Model file for the job. Use its own axes, mm. Face numbers are marked on the shaded views. A direction names the side the tool comes from. Give positions to 0.01 mm unless a question says otherwise; leave off trailing zeros. Order: outer loops, then holes, each group sorted by start corner. A loop starts at its lowest first (then second) coordinate and runs counter-clockwise, first axis right, second up. Notation, with made-up numbers: M 52.25,40 L 98.25,40 A22 ccw 98.25,60 Z; hole C -27,60.5 d7. An arc over 180 degrees is marked long. Return JSON: item names as keys, results as strings. Group by question number.
1. 3-axis set-ups, long thin cutter, end or side, ignore diameter. For the marked faces 1 and 2: which of +Z, -Z, +X, -X, +Y, -Y reach the whole face in a straight line?
2. Slice it at D-D on y = -3.5. List the corners of the cut face in (x, z).
3. Wall check: probe 1 along Y at (x, z) = (-11.5, 4.5); probe 2 along Y at (x, z) = (11, 2); probe 3 along Z at (x, y) = (-13, -3.5). Give the ranges that are in metal, low to high. Write a range as [from, to].
4. Pin check, flat tips, straight feed: pin 1 (1.5 mm diameter, centred on x = -15, y = -6, fed in from +Z); pin 2 (1.5 mm diameter, centred on y = -10.5, z = 33, fed in from +X). Stop position of each tip, or through.
5. Slice it at B-B on z = 17.5. List the corners of the cut face in (x, y).
6. Slice it at C-C on x = -11.5. List the corners of the cut face in (y, z), then the cut area to 3 significant figures.
7. Two-plate mould, pull along Y, no slides. Class the marked faces 3, 4 and 5: released by +Y, released by -Y, zero draft, split by the parting line, or undercut.
8. Slice it at A-A on x = 0. List the corners of the cut face in (y, z), then the cut area to 3 significant figures.
from build123d import *

# Parameters (mm, degrees)
SKETCH_1_W      = 5
SKETCH_1_H      = 28
SKETCH_1_W_2    = 28
SKETCH_1_R      = 1.5
EXTRUDE_1_DEPTH = 10
SKETCH_3_W      = 10
SKETCH_3_H      = 28
SKETCH_3_W_2    = 5
EXTRUDE_3_DEPTH = 6
FILLET_3_R      = 5
FILLET_4_R      = 2


with BuildPart() as part:
    # 草图1 → 凸台-拉伸1 (new body)
    # profile 1 of 2: a face of its own
    with BuildSketch(Plane.XY):
        with Locations((-16.5, 0)):
            Rectangle(SKETCH_1_W, SKETCH_1_H)
    # profile 2 of 2: a face of its own
    with BuildSketch(Plane.XY):
        Rectangle(SKETCH_1_W_2, SKETCH_1_H)
        Circle(SKETCH_1_R, mode=Mode.SUBTRACT)
        with Locations((11.5, -11.5)):
            Circle(SKETCH_1_R, mode=Mode.SUBTRACT)
        with Locations((-11.5, -11.5)):
            Circle(SKETCH_1_R, mode=Mode.SUBTRACT)
        with Locations((11.5, 11.5)):
            Circle(SKETCH_1_R, mode=Mode.SUBTRACT)
        with Locations((-11.5, 11.5)):
            Circle(SKETCH_1_R, mode=Mode.SUBTRACT)
    extrude(amount=EXTRUDE_1_DEPTH)

    # 草图3 → 凸台-拉伸3 (add)
    with BuildSketch(Plane.ZY.offset(19)):
        with Locations((5, 0)):
            Rectangle(SKETCH_3_W, SKETCH_3_H)
        with Locations((12.5, 0)):
            Rectangle(SKETCH_3_W_2, SKETCH_3_H)
        with BuildLine():
            Line((16.616116524, 12.383883476), (15, 14))
            Line((15, 14), (15, -14))
            Line((15, -14), (16.616116524, -12.383883476))
            ThreePointArc((16.616116524, -12.383883476), (16.616116524, -10.616116524), (18.383883476, -10.616116524))
            Line((18.383883476, -10.616116524), (27.232233047, -1.767766953))
            ThreePointArc((27.232233047, -1.767766953), (26.5, 0), (27.232233047, 1.767766953))
            Line((27.232233047, 1.767766953), (18.383883476, 10.616116524))
            ThreePointArc((18.383883476, 10.616116524), (16.616116524, 10.616116524), (16.616116524, 12.383883476))
        make_face()
        with BuildLine():
            Line((43, 14), (15, 14))
            Line((15, 14), (16.616116524, 12.383883476))
            ThreePointArc((16.616116524, 12.383883476), (17.97835429, 12.654849416), (18.75, 11.5))
            ThreePointArc((18.75, 11.5), (18.654849416, 11.02164571), (18.383883476, 10.616116524))
            Line((18.383883476, 10.616116524), (27.232233047, 1.767766953))
            ThreePointArc((27.232233047, 1.767766953), (29, 2.5), (30.767766953, 1.767766953))
            Line((30.767766953, 1.767766953), (39.616116524, 10.616116524))
            ThreePointArc((39.616116524, 10.616116524), (39.616116524, 12.383883476), (41.383883476, 12.383883476))
            Line((41.383883476, 12.383883476), (43, 14))
        make_face()
        with BuildLine():
            Line((43, -14), (43, 14))
            Line((43, 14), (41.383883476, 12.383883476))
            ThreePointArc((41.383883476, 12.383883476), (41.654849416, 11.97835429), (41.75, 11.5))
            ThreePointArc((41.75, 11.5), (40.97835429, 10.345150584), (39.616116524, 10.616116524))
            Line((39.616116524, 10.616116524), (30.767766953, 1.767766953))
            ThreePointArc((30.767766953, 1.767766953), (31.309698831, 0.956708581), (31.5, 0))
            ThreePointArc((31.5, 0), (31.309698831, -0.956708581), (30.767766953, -1.767766953))
            Line((30.767766953, -1.767766953), (39.616116524, -10.616116524))
            ThreePointArc((39.616116524, -10.616116524), (40.97835429, -10.345150584), (41.75, -11.5))
            ThreePointArc((41.75, -11.5), (41.654849416, -11.97835429), (41.383883476, -12.383883476))
            Line((41.383883476, -12.383883476), (43, -14))
        make_face()
        with BuildLine():
            Line((16.616116524, -12.383883476), (15, -14))
            Line((15, -14), (43, -14))
            Line((43, -14), (41.383883476, -12.383883476))
            ThreePointArc((41.383883476, -12.383883476), (39.616116524, -12.383883476), (39.616116524, -10.616116524))
            Line((39.616116524, -10.616116524), (30.767766953, -1.767766953))
            ThreePointArc((30.767766953, -1.767766953), (29, -2.5), (27.232233047, -1.767766953))
            Line((27.232233047, -1.767766953), (18.383883476, -10.616116524))
            ThreePointArc((18.383883476, -10.616116524), (18.654849416, -11.02164571), (18.75, -11.5))
            ThreePointArc((18.75, -11.5), (17.97835429, -12.654849416), (16.616116524, -12.383883476))
        make_face()
    extrude(amount=EXTRUDE_3_DEPTH)

    # 圆角3
    fillet_3_edges = [part.edges().sort_by_distance(p)[0] for p in [
        (-25, 0, 0),
    ]]
    fillet(fillet_3_edges, radius=FILLET_3_R)

    # 圆角4
    fillet_4_edges = [part.edges().sort_by_distance(p)[0] for p in [
        (-19, 0, 10),
    ]]
    fillet(fillet_4_edges, radius=FILLET_4_R)


solid = part.part
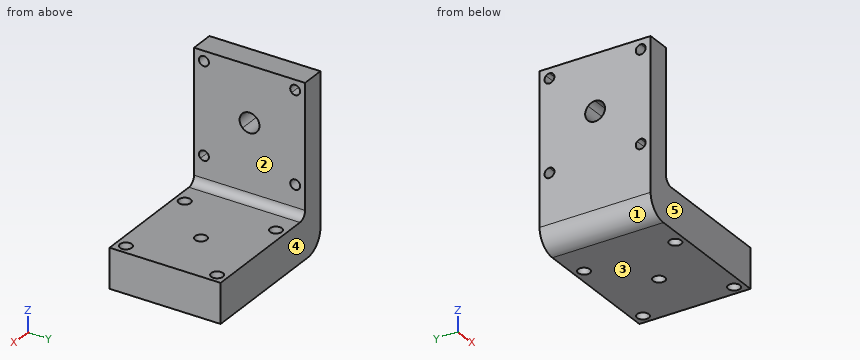
Result:
{
 "1": {"face 1": "-Z, -X, +Y, -Y", "face 2": "+Z, +X, +Y, -Y"},
 "2": {"outline": "M -25,5 A5 ccw -20,0 L 14,0 L 14,10 L -17,10 A2 cw -19,12 L -19,43 L -25,43 Z"},
 "3": {"probe 1": "y = [-14, -13], [-10, 10], [13, 14]", "probe 2": "y = [-14, -12.91], [-10.09, 10.09], [12.91, 14]", "probe 3": "z = [0, 10]"},
 "4": {"pin 1": "stops at z = 10", "pin 2": "stops at x = -19"},
 "5": {"outline": "M -25,-14 L -19,-14 L -19,-12.75 L -25,-12.75 Z; M -25,-10.25 L -19,-10.25 L -19,10.25 L -25,10.25 Z; M -25,12.75 L -19,12.75 L -19,14 L -25,14 Z"},
 "6": {"outline": "M -14,0 L -13,0 L -13,10 L -14,10 Z; M -10,0 L 10,0 L 10,10 L -10,10 Z; M 13,0 L 14,0 L 14,10 L 13,10 Z", "area": "220 mm2"},
 "7": {"face 3": "zero draft", "face 4": "released by +Y", "face 5": "released by -Y"},
 "8": {"outline": "M -14,0 L -1.5,0 L -1.5,10 L -14,10 Z; M 1.5,0 L 14,0 L 14,10 L 1.5,10 Z", "area": "250 mm2"}
}
